For this review, take the finished solid that the model builds, in its own axes (mm). Face numbers are marked on the shaded views. A direction names the side the tool comes from. Coordinates: 2 decimals unless noted, no trailing zeros. Loops run counter-clockwise (first coordinate to the right, second up) from the corner with the lowest first, then second, coordinate; pieces in that order, holes last. Notation, with made-up numbers: (77.5, 57.25) - (133.5, 57.25) arc R14 ccw to (133.5, 70.25) - close; hole circle Ø3 at (49.25, -22). An arc over 180 degrees is marked (long way). Answer as a JSON object with one key per item and string values. Group by question number.
Item 1: We need section C-C (y = 20). Give the boundary of the cut face in (x, z).
Item 2: Tool access review of the marked faces 1 and 2: name each direction out of +Z, -Z, +X, -X, +Y, -Y from which nothing blocks a thin tool from reaching the whole face with its end or side.
Item 3: Clearance check with flat-ended pins moving along their axes: pin 1 (6.5 mm diameter, centred on x = -56.5, y = 24.5, fed in from -Z); pin 2 (5.5 mm diameter, centred on y = 25, z = -50, fed in from -X); pin 3 (3.5 mm diameter, centred on y = 0, z = -55, fed in from -X). State where each tip first meets the part, or that it passes through.
Item 4: To check wall thickness, follow line 1 (Y direction, x = -55, z = -25); line 2 (X direction, y = 27, z = -36.5); line 3 (X direction, y = -19.5, z = -34.5). State the ranges of each line that lie inside material, in increasing order.
Item 5: We need section D-D (z = -55). Give the boundary of the cut face in (x, y).
Item 6: Mouldability with a two-part tool opening along X and no side actions: class the marked faces 3, 4, 5 and 6 as released by +X, released by -X, zero draft, split by the parting line, or undercut.
Item 7: We need section A-A (x = -36.5). Give the boundary of the cut face in (y, z).
Item 8: We need section B-B (z = -45). Give the boundary of the cut face in (x, y).
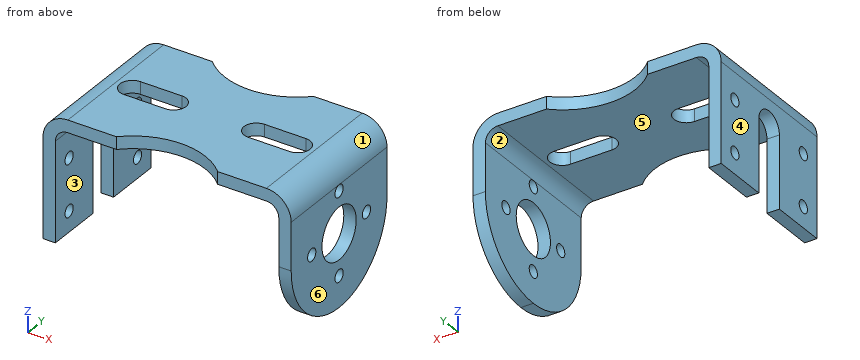
from build123d import *

# Parameters (mm, degrees)
SKETCH1_W                    = 108
SKETCH1_H                    = 70
BASE_FLANGE1_DEPTH           = 6
EDGE_FLANGE1_STRIP_W         = 36
EDGE_FLANGE1_STRIP_H         = 6
EDGE_FLANGE1_STRIP_CUT_DEPTH = 70
EDGE_FLANGE1_DEPTH           = 70
EDGE_FLANGE2_STRIP_W         = 36
EDGE_FLANGE2_STRIP_H         = 6
EDGE_FLANGE2_STRIP_CUT_DEPTH = 70
EDGE_FLANGE2_DEPTH           = 70
FILLET1_R                    = 35
CUT_EXTRUDE1_DEPTH           = 6
SKETCH15_R                   = 3
CUT_EXTRUDE2_DEPTH           = 7
LPATTERN1_COUNT              = 2
LPATTERN1_PITCH              = 50
CUT_EXTRUDE3_DEPTH           = 7
LPATTERN2_COUNT              = 2
LPATTERN2_PITCH              = 60
CUT_EXTRUDE4_DEPTH           = 8
SKETCH27_R                   = 3
CUT_EXTRUDE6_DEPTH           = 8
HOLE2_START                  = 54
HOLE2_OUTLINE_R              = 12.5
HOLE2_DEPTH                  = 6


# Read off the part's stored shape, not the designer's step: Hole2
# Sheet-metal steps are written as plain solids
with BuildPart() as part:
    # Sketch1 → Base-Flange1 (new body)
    with BuildSketch(Plane.XY):
        Rectangle(SKETCH1_W, SKETCH1_H)
    extrude(amount=-BASE_FLANGE1_DEPTH)

    # Edge-Flange1 strip (across the edge) → Edge-Flange1 strip cut (cut)
    with BuildSketch(Plane(origin=(54, 35, -6), x_dir=(-1, 0, 0), z_dir=(0, -1, 0))):
        with Locations((-12, -3)):
            Rectangle(EDGE_FLANGE1_STRIP_W, EDGE_FLANGE1_STRIP_H)
    extrude(amount=EDGE_FLANGE1_STRIP_CUT_DEPTH, mode=Mode.SUBTRACT)

    # Edge-Flange1 section (across the edge) → Edge-Flange1 (add)
    with BuildSketch(Plane(origin=(54, 35, -6), x_dir=(-1, 0, 0), z_dir=(0, -1, 0))):
        with BuildLine():
            Line((-6, 6), (-6, 64))
            Line((-6, 64), (0, 64))
            Line((0, 64), (0, 6))
            ThreePointArc((0, 6), (1.757359313, 1.757359313), (6, 0))
            Line((6, 0), (6, -6))
            ThreePointArc((6, -6), (-2.485281374, -2.485281374), (-6, 6))
        make_face()
    extrude(amount=EDGE_FLANGE1_DEPTH)

    # Edge-Flange2 strip (across the edge) → Edge-Flange2 strip cut (cut)
    with BuildSketch(Plane(origin=(-54, -35, -6), x_dir=(1, 0, 0), z_dir=(0, 1, 0))):
        with Locations((-12, -3)):
            Rectangle(EDGE_FLANGE2_STRIP_W, EDGE_FLANGE2_STRIP_H)
    extrude(amount=EDGE_FLANGE2_STRIP_CUT_DEPTH, mode=Mode.SUBTRACT)

    # Edge-Flange2 section (across the edge) → Edge-Flange2 (add)
    with BuildSketch(Plane(origin=(-54, -35, -6), x_dir=(1, 0, 0), z_dir=(0, 1, 0))):
        with BuildLine():
            Line((-6, 6), (-6, 54))
            Line((-6, 54), (0, 54))
            Line((0, 54), (0, 6))
            ThreePointArc((0, 6), (1.757359313, 1.757359313), (6, 0))
            Line((6, 0), (6, -6))
            ThreePointArc((6, -6), (-2.485281374, -2.485281374), (-6, 6))
        make_face()
    extrude(amount=EDGE_FLANGE2_DEPTH)

    # Fillet1
    fillet1_edges = [part.edges().sort_by_distance(p)[0] for p in [
        (57, -35, -70),
        (57, 35, -70),
    ]]
    fillet(fillet1_edges, radius=FILLET1_R - 0.0001)  # a hair under: the kernel refuses the full size

    # Sketch14 → Cut-Extrude1 (cut)
    with BuildSketch(Plane.ZY.offset(60)):
        with BuildLine():
            Line((-60, 7.5), (-60, -7.5))
            Line((-60, -7.5), (-25, -7.5))
            ThreePointArc((-25, -7.5), (-17.5, 0), (-25, 7.5))
            Line((-25, 7.5), (-60, 7.5))
        make_face()
    extrude(amount=-CUT_EXTRUDE1_DEPTH, mode=Mode.SUBTRACT)

    # Sketch15 → Cut-Extrude2 (cut)
    with BuildSketch(Plane.ZY.offset(60)):
        with Locations((-50, 25)):
            Circle(SKETCH15_R)
        with Locations((-25, 25)):
            Circle(SKETCH15_R)
    cut_extrude2 = extrude(amount=-CUT_EXTRUDE2_DEPTH, mode=Mode.SUBTRACT)

    # LPattern1: Cut-Extrude2 ×2
    with Locations(*[(0, -i * LPATTERN1_PITCH, 0) for i in range(1, LPATTERN1_COUNT)]):
        add(cut_extrude2, mode=Mode.SUBTRACT)

    # Sketch16 → Cut-Extrude3 (cut)
    with BuildSketch(Plane(origin=(0, 0, -6), x_dir=(-1, 0, 0), z_dir=(0, 0, -1))):
        with BuildLine():
            Line((-40, 6), (-20, 6))
            ThreePointArc((-20, 6), (-14, 0), (-20, -6))
            Line((-20, -6), (-40, -6))
            ThreePointArc((-40, -6), (-46, 0), (-40, 6))
        make_face()
    cut_extrude3 = extrude(amount=-CUT_EXTRUDE3_DEPTH, mode=Mode.SUBTRACT)

    # LPattern2: Cut-Extrude3 ×2
    with Locations(*[(-i * LPATTERN2_PITCH, 0, 0) for i in range(1, LPATTERN2_COUNT)]):
        add(cut_extrude3, mode=Mode.SUBTRACT)

    # Sketch18 → Cut-Extrude4 (cut)
    with BuildSketch(Plane(origin=(0, 0, -6), x_dir=(-1, 0, 0), z_dir=(0, 0, -1))):
        with BuildLine():
            Line((24.494897428, -35), (-24.494897428, -35))
            ThreePointArc((-24.494897428, -35), (0, -25), (24.494897428, -35))
        make_face()
    cut_extrude4 = extrude(amount=-CUT_EXTRUDE4_DEPTH, mode=Mode.SUBTRACT)

    # Sketch27 → Cut-Extrude6 (cut)
    with BuildSketch(Plane(origin=(60, 0, 0), x_dir=(0, 0, -1), z_dir=(1, 0, 0))):
        with Locations((55, 0)):
            Circle(SKETCH27_R)
        with Locations((35, 20)):
            Circle(SKETCH27_R)
        with Locations(Location((15, 0, 0), (0, 0, 180))):
            Circle(SKETCH27_R)
        with Locations((35, -20)):
            Circle(SKETCH27_R)
    extrude(amount=-CUT_EXTRUDE6_DEPTH, mode=Mode.SUBTRACT)

    # Hole2 outline → Hole2 (cut)
    with BuildSketch(Plane.YZ.offset(HOLE2_START)):
        with Locations((0, -35)):
            Circle(HOLE2_OUTLINE_R)
    extrude(amount=HOLE2_DEPTH, mode=Mode.SUBTRACT)

    # Mirror2: Cut-Extrude4 across plane
    add(cut_extrude4.mirror(Plane.ZX), mode=Mode.SUBTRACT)


solid = part.part
Check sheet entries:
{
 "1": {"outline": "(-60, -60) - (-54, -60) - (-54, -12) arc R6 cw to (-48, -6) - (48, -6) arc R6 cw to (54, -12) - (54, -32) - (60, -32) - (60, -12) arc R12 ccw to (48, 0) - (-48, 0) arc R12 ccw to (-60, -12) - close; (54, -63.72) - (60, -63.72) - (60, -38) - (54, -38) - close"},
 "2": {"face 1": "+Z, +X, +Y, -Y", "face 2": "-Z, +Y, -Y"},
 "3": {"pin 1": "stops at z = -60", "pin 2": "stops at x = 54", "pin 3": "passes through"},
 "4": {"line 1": "y = -35 to -28, -22 to -7.5, 7.5 to 22, 28 to 35", "line 2": "x = -60 to -54, 54 to 60", "line 3": "x = -60 to -54"},
 "5": {"outline": "(-60, -35) - (-54, -35) - (-54, -7.5) - (-60, -7.5) - close; (-60, 7.5) - (-54, 7.5) - (-54, 35) - (-60, 35) - close; (54, -28.72) - (60, -28.72) - (60, -3) - (54, -3) - close; (54, 3) - (60, 3) - (60, 28.72) - (54, 28.72) - close"},
 "6": {"face 3": "undercut", "face 4": "released by -X", "face 5": "undercut", "face 6": "released by +X"},
 "7": {"outline": "(-35, -6) - (-6, -6) - (-6, 0) - (-35, 0) - close; (6, -6) - (35, -6) - (35, 0) - (6, 0) - close"},
 "8": {"outline": "(-60, -35) - (-54, -35) - (-54, -7.5) - (-60, -7.5) - close; (-60, 7.5) - (-54, 7.5) - (-54, 35) - (-60, 35) - close; (54, -33.54) - (60, -33.54) - (60, -7.5) - (54, -7.5) - close; (54, 7.5) - (60, 7.5) - (60, 33.54) - (54, 33.54) - close"}
}
